The model under review builds one solid part; all positions refer to its coordinate system, in mm. Face numbers are marked on the shaded views. A direction names the side the tool comes from. Coordinates: 2 decimals unless noted, no trailing zeros. Order: outer loops, then holes, each group sorted by start corner. A loop starts at its lowest first (then second) coordinate and runs counter-clockwise, first axis right, second up. Notation, with made-up numbers: (32, 11) -> (60, 11) arc R25 ccw to (60, 49) -> close; hole circle Ø6 at (24.25, -38). An arc over 180 degrees is marked (long way). Put each result on its own line as item: value.
Autodesk Fusion 360 part; units mm, degrees
sketch "Sketch1" plane through (0, 0, 0) normal (0, 1, 0) x (1, 0, 0)
  line L0 (0, 0) -> (30, 0)
  line L1 (30, 0) -> (30, -18)
  line L2 (30, -18) -> (0, -18)
  line L3 (0, -18) -> (0, 0)
  dimension "d1" = 30
  dimension "d2" = 18
extrude "Extrude1" add sketch "Sketch1" along normal blind 9.6
sketch "Sketch2" plane through (0, 9.6, 0) normal (0, 1, 0) x (-1, 0, 0)
  line L0 (0, 18) -> (-30, 18)
  line L1 (-30, 18) -> (-30, 0)
  line L2 (-30, 0) -> (0, 0)
  line L3 (0, 0) -> (0, 18)
  circle A0 centre (-3.9, 3.9) radius 2.5
  dimension "d5" = 5
  dimension "d6" = 3.9
  dimension "d7" = 3.9
extrude "Extrude2" add sketch "Sketch2" along normal blind 1.7 contours A0
pattern_linear "R-Pattern1" count 3 spacing 10 along (1, 0, 0) count 2 spacing 8 along (0, 0, 1) of "Extrude2"
shell "Shell1" thickness 1.5 removed faces 1 at (10, 0, 6)
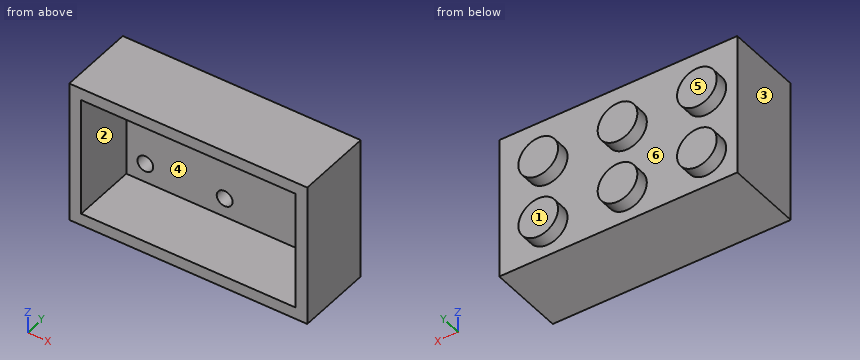
Item 1: Consider section A-A on y = 1. Write out the cut boundary in (x, z), and give its area (3 significant figures).
Answers below:
outline: (0, 0) -> (30, 0) -> (30, 18) -> (0, 18) -> close; hole (1.5, 1.5) -> (28.5, 1.5) -> (28.5, 16.5) -> (1.5, 16.5) -> close
area: 135 mm^2
Item 2: For pin 1 Ø10 at (x, z) = (16.5, 6) entering from +Y; pin 2 Ø2.5 at (x, z) = (13.9, 11.9) entering from -Y; pin 3 Ø0.6 at (x, z) = (24, 4) entering from -Y, all flat-tipped, find the tip position at first contact; note any pin that passes through.
Answers below:
pin 1: y = 11.3
pin 2: y = 8.1
pin 3: y = 9.8
Item 3: For the marked faces 4, 5 and 6, list the 3-axis set-ups (+Z, -Z, +X, -X, +Y, -Y) from which the entire face can be reached by the end or side of a thin tool; tool diameter is ignored.
Answers below:
face 4: -Y
face 5: +Z, -Z, +X, -X, +Y
face 6: +Y
Item 4: Consider section C-C on x = 13.9. Write out the cut boundary in (y, z), and give its area (3 significant figures).
Answers below:
outline: (0, 0) -> (9.6, 0) -> (9.6, 1.4) -> (11.3, 1.4) -> (11.3, 6.4) -> (9.6, 6.4) -> (9.6, 9.4) -> (11.3, 9.4) -> (11.3, 14.4) -> (9.6, 14.4) -> (9.6, 18) -> (0, 18) -> (0, 16.5) -> (8.1, 16.5) -> (8.1, 12.9) -> (9.8, 12.9) -> (9.8, 10.9) -> (8.1, 10.9) -> (8.1, 4.9) -> (9.8, 4.9) -> (9.8, 2.9) -> (8.1, 2.9) -> (8.1, 1.5) -> (0, 1.5) -> close
area: 61.5 mm^2
Item 5: For line 1 (X direction, y = 9.15, z = 11.9); line 2 (Z direction, x = 13.9, y = 8.85); line 3 (Z direction, x = 5.25, y = 7.5), list the stretches that pass through material, from the lowest coordinate up. Write a range as from..to.
Answers below:
line 1: 0..2.9, 4.9..12.9, 14.9..22.9, 24.9..30
line 2: 0..2.9, 4.9..10.9, 12.9..18
line 3: 0..1.5, 16.5..18
Item 6: Mouldability with a two-part tool opening along X and no side actions: class the marked faces 1, 2 and 3 as +X half, -X half, draft (parallel to the pull), parting line (faces both ways), or undercut.
Answers below:
face 1: draft
face 2: undercut
face 3: -X half
Item 7: Consider section D-D on z = 15.5. Write out the cut boundary in (x, y), and give its area (3 significant figures).
Answers below:
outline: (0, 0) -> (1.5, 0) -> (1.5, 8.1) -> (28.5, 8.1) -> (28.5, 0) -> (30, 0) -> (30, 9.6) -> (0, 9.6) -> close
area: 69.3 mm^2
